Input: part model. Units: mm. Frame: model coordinates. A direction names the side the tool comes from. Round coordinates to 2 decimals unless told otherwise and drop trailing zeros. Loops run counter-clockwise (first coordinate to the right, second up) from the corner with the lowest first, then second, coordinate; pieces in that order, holes last.
1) Ray query, line 1 along Y through (x, z) = (-7.5, 4.75); line 2 along Y through (x, z) = (-4.5, 1.25); line 3 along X through (y, z) = (-4.5, 2.25) (3 decimals). Return the intervals inside material, ascending.
2) Section A-A, the plane x = -39. Return loops of the section in (y, z), and give its area (3 significant figures).
3) Draft query along Y for faces 5 (the face through (-58.331, 0.986, 9.398)), 6 (the face through (-45.6, -10.2, 11)), 7 (the face through (-20, 15, 5)). Return one class per face: pulls with the +Y half, pulls with the -Y half, needs draft (parallel to the pull), parting line crosses it, or undercut.
4) Access query for faces 1 (the face through (-30.345, 8, 3)), 2 (the face through (-15.655, 0, 1)), 3 (the face through (21, 5.5, 3)), 4 (the face through (1, 0, 2)). Directions: +Z, -Z, +X, -X, +Y, -Y. A direction counts if a zero-diameter tool reaches every point of the face in a straight line with its end or side. Return the directions, or none.
5) First-contact query: pin 1 (1 mm diameter, centred on y = -11, z = 3, fed in from -X) (3 decimals); pin 2 (3 mm diameter, centred on x = 6.5, y = -8, fed in from +Z); pin 3 (10 mm diameter, centred on x = 10, y = 1, fed in from +Z); pin 4 (2.5 mm diameter, centred on x = 21.345, y = -11, fed in from +Z). Flat tips, straight axial feed; report the tip coordinate or a pass-through.
6) Section B-B, the plane y = -11. Return loops of the section in (x, z) (3 decimals).
Solid Edge part; units mm, degrees
sketch "Sketch1" plane through (0, 0, 0) normal (0, 0, 1) x (1, 0, 0)
  line L0 (-25.345, -15) -> (25.345, -15)
  line L1 (25.345, -15) -> (25.345, 15)
  line L2 (25.345, 15) -> (-25.345, 15)
  line L3 (-25.345, 15) -> (-25.345, -15)
  dimension "D1" = 25.345
  dimension "D2" = 25.345
extrude "Protrusion1" add sketch "Sketch1" along normal blind 6
sketch "Sketch2" plane through (0, 0, 6) normal (0, 0, 1) x (1, 0, 0)
  line L0 (-15.655, 6.25) -> (17.345, 6.25)
  line L1 (17.345, 6.25) -> (17.345, -6.25)
  line L2 (17.345, -6.25) -> (-15.655, -6.25)
  line L3 (-15.655, -6.25) -> (-15.655, 6.25)
  dimension "D1" = 15.655
  dimension "D2" = 17.345
extrude "Utskärning_för_batteriet" cut sketch "Sketch2" against normal blind 4
hole "Hole1" at (21.345, 11, 6) direction (0, 0, -1) diameter 4 end up to next
hole "Hole2" at (21.345, -11, 6) direction (0, 0, -1) diameter 4 end up to next
hole "Hole3" at (-18.655, 11, 6) direction (0, 0, -1) diameter 4 end up to next
hole "Hole4" at (-18.655, -11, 6) direction (0, 0, -1) diameter 4 end up to next
sketch "Sketch3" plane through (-0.5, -15, 3) normal (0, -1, 0) x (1, 0, 0)
  line L0 (-24.845, 3) -> (-24.845, 8)
  line L1 (-24.845, 8) -> (-64.845, 8)
  line L2 (-64.845, 8) -> (-64.845, 2)
  line L3 (-64.845, 2) -> (-29.845, 2)
  line L4 (-29.845, 2) -> (-29.845, -3)
  line L5 (-29.845, -3) -> (-24.845, -3)
  line L6 (-24.845, -3) -> (-24.845, 3)
  dimension "D1" = 24.845
  dimension "D2" = 64.845
  dimension "D3" = 64.845
  dimension "D4" = 29.845
extrude "Protrusion2" add sketch "Sketch3" against normal up to vertex (30 mm away)
sketch "Sketch4" plane through (0, 0, 6) normal (0, 0, 1) x (0, -1, 0)
  line L0 (-5.5, 23.345) -> (5.5, 23.345)
  line L1 (5.5, 23.345) -> (5.5, 19.345)
  line L2 (5.5, 19.345) -> (-5.5, 19.345)
  line L3 (-5.5, 19.345) -> (-5.5, 23.345)
  line L4 (-13, 17.265) -> (-9, 17.265)
  line L5 (-9, 17.265) -> (-9, -13.735)
  line L6 (-9, -13.735) -> (-13, -13.735)
  line L7 (-13, -13.735) -> (-13, 17.265)
  line L8 (9, 17.265) -> (13, 17.265)
  line L9 (13, 17.265) -> (13, -13.735)
  line L10 (13, -13.735) -> (9, -13.735)
  line L11 (9, -13.735) -> (9, 17.265)
  line L12 (-10, -57.345) -> (10, -57.345)
  line L13 (10, -57.345) -> (10, -33.345)
  line L14 (10, -33.345) -> (-10, -33.345)
  line L15 (-10, -33.345) -> (-10, -57.345)
  dimension "D1" = 5.5
  dimension "D2" = 5.5
extrude "Cutout1" cut sketch "Sketch4" along normal through all and the other way through all
sketch "Sketch5" plane through (0, 0, 6) normal (0, 0, 1) x (0, -1, 0)
  line L0 (-2.76, -15.655) -> (-2.76, -33.345)
  line L1 (-2.76, -33.345) -> (2.76, -33.345)
  line L2 (2.76, -33.345) -> (2.76, -15.655)
  line L3 (2.76, -15.655) -> (-2.76, -15.655)
  dimension "D1" = 2.76
extrude "Cutout2" cut sketch "Sketch5" along normal through all and the other way through all
fillet "Avrundningar_1" radius 1 35 edges at (25.345, 15, 3) (17.345, 6.25, 4) (25.345, -15, 3) (17.345, -6.25, 4) (25.345, 0, 0) (-15.655, -6.25, 4) (-15.655, 6.25, 4) (-2.5, -15, 0) (-30.345, 8.88, 0) (-30.345, -8.88, 0) (-30.345, -15, 2.5) (-30.345, 15, 2.5) (-2.5, 15, 0) (-15.655, 2.76, 4) (-15.655, -2.76, 4) (-33.345, 10, 8) (-33.345, -10, 8) (-57.345, 10, 8) (-57.345, -10, 8) (-33.345, 2.76, 8) (-33.345, -2.76, 8) (-13.735, 13, 3) (-13.735, 9, 3) (-13.735, -13, 3) (-13.735, -9, 3) (17.265, 13, 3) (17.265, -9, 3) (17.265, 9, 3) (23.345, -5.5, 3) (17.265, -13, 3) (23.345, 5.5, 3) (19.345, -5.5, 3) (19.345, 5.5, 3) (-25.345, 8.88, 11) (-25.345, -8.88, 11)
sketch "Sketch6" plane through (-57.345, 0, 6) normal (1, 0, 0) x (0, -1, 0)
  line L0 (0, -4.5004) -> (-2, -2.2644)
  line L1 (-2, -2.2644) -> (-0.5, -2.2644)
  line L2 (-0.5, -2.2644) -> (-0.5, 0.2356)
  line L3 (-0.5, 0.2356) -> (0.5, 0.2356)
  line L4 (0.5, 0.2356) -> (0.5, -2.2644)
  line L5 (0.5, -2.2644) -> (2, -2.2644)
  line L6 (2, -2.2644) -> (0, -4.5004)
  dimension "D1" = 0.5
  dimension "D2" = 2
  dimension "D3" = 0.5
extrude "Utskärning_pil" cut sketch "Sketch6" against normal blind 2
Final values:
1. line 1: y = -15 to -13, -9 to -6.25, 6.25 to 9, 13 to 15
1. line 2: y = -15 to -13, -9 to 9, 13 to 15
1. line 3: x = -30.345 to -15.655, 17.345 to 19.345, 23.345 to 25.345
2. outline: (-15, 5) - (-10, 5) - (-10, 11) - (-15, 11) - close; (10, 5) - (15, 5) - (15, 11) - (10, 11) - close
2. area: 60.0 mm2
3. face 5: undercut
3. face 6: needs draft
3. face 7: pulls with the +Y half
4. face 1: -Z, -X, +Y, -Y
4. face 2: +Z, -Z, -X
4. face 3: +Z, -Z
4. face 4: +Z
5. pin 1: stops at x = -30.345
5. pin 2: stops at z = 6
5. pin 3: stops at z = 2
5. pin 4: passes through
6. outline: (-65.345, 5) - (-30.345, 5) - (-30.345, 1) arc R1 ccw to (-29.345, 0) - (-20.655, 0) - (-20.655, 6) - (-25.345, 6) - (-25.345, 10) arc R1 ccw to (-26.345, 11) - (-65.345, 11) - close; (-16.655, 0) - (-13.735, 0) - (-13.735, 6) - (-16.655, 6) - close; (17.265, 0) - (19.345, 0) - (19.345, 6) - (17.265, 6) - close; (23.345, 0) - (24.345, 0) arc R1 ccw to (25.345, 1) - (25.345, 6) - (23.345, 6) - close
